from build123d import *

# Parameters (mm, degrees)
F1_DEPTH = 65
F2_DEPTH = 14
F3_DEPTH = 14
F4_R     = 1
F5_DEPTH = 14


# Not quite as in the source:
# - a feature names something its author has since deleted; it is built from what else it names


with BuildPart() as f1:
    # F0 (on Top) → F1 (new body)
    with BuildSketch(Plane.XY):
        with BuildLine():
            ThreePointArc((0, -3), (2.1213203436, -2.1213203436), (3, 0))
            Line((3, 0), (0, 0))
            Line((0, 0), (0, -3))
        make_face()
        with BuildLine():
            Line((0, 0), (3, 0))
            ThreePointArc((3, 0), (2.1213203436, 2.1213203436), (0, 3))
            Line((0, 3), (0, 0))
        make_face()
        with BuildLine():
            Line((0, 0), (0, 3))
            ThreePointArc((0, 3), (-2.1213203436, 2.1213203436), (-3, 0))
            Line((-3, 0), (0, 0))
        make_face()
        with BuildLine():
            ThreePointArc((-3, 0), (-2.1213203436, -2.1213203436), (0, -3))
            Line((0, -3), (0, 0))
            Line((0, 0), (-3, 0))
        make_face()
    extrude(amount=F1_DEPTH)



with BuildPart() as f2:
    # F0 (on Top) → F2 (new body)
    with BuildSketch(Plane.XY):
        with BuildLine():
            ThreePointArc((-4.8989794856, 3), (-3.8729833462, 7.1622776602), (0, 9))
            Line((0, 9), (0, 12.5))
            ThreePointArc((0, 12.5), (-0.545120999, 12.4881080671), (-1.0892047912, 12.4524548954))
            ThreePointArc((-1.0892047912, 12.4524548954), (-8.8388347648, 8.8388347648), (-12.4524548954, 1.0892047912))
            ThreePointArc((-12.4524548954, 1.0892047912), (-12.4881080671, 0.545120999), (-12.5, 0))
            Line((-12.5, 0), (-4.8989794856, 0))
            Line((-4.8989794856, 0), (-4.8989794856, 3))
        make_face()
        with BuildLine():
            Line((0, -12.5), (0, -9))
            ThreePointArc((0, -9), (-3.8729833462, -7.1622776602), (-4.8989794856, -3))
            Line((-4.8989794856, -3), (-4.8989794856, 0))
            Line((-4.8989794856, 0), (-12.5, 0))
            ThreePointArc((-12.5, 0), (-8.8388347648, -8.8388347648), (0, -12.5))
        make_face()
        with BuildLine():
            Line((12.5, 0), (4.8989794856, 0))
            Line((4.8989794856, 0), (4.8989794856, -3))
            ThreePointArc((4.8989794856, -3), (3.8729833462, -7.1622776602), (0, -9))
            Line((0, -9), (0, -12.5))
            ThreePointArc((0, -12.5), (0.545120999, -12.4881080671), (1.0892047912, -12.4524548954))
            ThreePointArc((1.0892047912, -12.4524548954), (8.8388347648, -8.8388347648), (12.4524548954, -1.0892047912))
            ThreePointArc((12.4524548954, -1.0892047912), (12.4881080671, -0.545120999), (12.5, 0))
        make_face()
        with BuildLine():
            Line((4.8989794856, 3), (4.8989794856, 0))
            Line((4.8989794856, 0), (12.5, 0))
            ThreePointArc((12.5, 0), (8.8388347648, 8.8388347648), (0, 12.5))
            Line((0, 12.5), (0, 9))
            ThreePointArc((0, 9), (3.8729833462, 7.1622776602), (4.8989794856, 3))
        make_face()
    extrude(amount=F2_DEPTH)


with BuildPart() as f1_1:
    add(f1.part)

    add(f2.part)  # F2#2 merges F2
    # F0 (on Top) → F2, piece 2 (join)
    with BuildSketch(Plane.XY):
        with BuildLine():
            ThreePointArc((-3, 0), (-2.1213203436, 2.1213203436), (0, 3))
            Line((0, 3), (-4.8989794856, 3))
            ThreePointArc((-4.8989794856, 3), (-4.2247448714, 1.3257653858), (-3, 0))
        make_face()
        with BuildLine():
            ThreePointArc((0, 3), (2.1213203436, 2.1213203436), (3, 0))
            ThreePointArc((3, 0), (4.2247448714, 1.3257653858), (4.8989794856, 3))
            Line((4.8989794856, 3), (0, 3))
        make_face()
        with BuildLine():
            ThreePointArc((4.8989794856, -3), (4.2247448714, -1.3257653858), (3, 0))
            ThreePointArc((3, 0), (2.1213203436, -2.1213203436), (0, -3))
            Line((0, -3), (4.8989794856, -3))
        make_face()
        with BuildLine():
            Line((-4.8989794856, -3), (0, -3))
            ThreePointArc((0, -3), (-2.1213203436, -2.1213203436), (-3, 0))
            ThreePointArc((-3, 0), (-4.2247448714, -1.3257653858), (-4.8989794856, -3))
        make_face()
    extrude(amount=F2_DEPTH)

    # F0 (on Top) → F3 (join)
    with BuildSketch(Plane.XY):
        with BuildLine():
            Line((20, 0), (12.5, 0))
            ThreePointArc((12.5, 0), (14.2975101103, -0.811390688), (16.25, -1.0892047912))
            ThreePointArc((16.25, -1.0892047912), (18.2024898897, -0.811390688), (20, 0))
        make_face()
        with BuildLine():
            ThreePointArc((-1.0892047912, 16.25), (-0.811390688, 14.2975101103), (0, 12.5))
            Line((0, 12.5), (0, 20))
            ThreePointArc((0, 20), (-0.811390688, 18.2024898897), (-1.0892047912, 16.25))
        make_face()
        with BuildLine():
            Line((-20, 0), (-12.5, 0))
            ThreePointArc((-12.5, 0), (-14.2975101103, 0.811390688), (-16.25, 1.0892047912))
            ThreePointArc((-16.25, 1.0892047912), (-18.2024898897, 0.811390688), (-20, 0))
        make_face()
        with BuildLine():
            ThreePointArc((1.0892047912, -16.25), (0.811390688, -14.2975101103), (0, -12.5))
            Line((0, -12.5), (0, -20))
            ThreePointArc((0, -20), (0.811390688, -18.2024898897), (1.0892047912, -16.25))
        make_face()
        with BuildLine():
            ThreePointArc((16.25, -1.0892047912), (14.2975101103, -0.811390688), (12.5, 0))
            ThreePointArc((12.5, 0), (12.4881080671, -0.545120999), (12.4524548954, -1.0892047912))
            Line((12.4524548954, -1.0892047912), (16.25, -1.0892047912))
        make_face()
        with BuildLine():
            ThreePointArc((-1.0892047912, 12.4524548954), (-0.545120999, 12.4881080671), (0, 12.5))
            ThreePointArc((0, 12.5), (-0.811390688, 14.2975101103), (-1.0892047912, 16.25))
            Line((-1.0892047912, 16.25), (-1.0892047912, 12.4524548954))
        make_face()
        with BuildLine():
            ThreePointArc((-16.25, 1.0892047912), (-14.2975101103, 0.811390688), (-12.5, 0))
            ThreePointArc((-12.5, 0), (-12.4881080671, 0.545120999), (-12.4524548954, 1.0892047912))
            Line((-12.4524548954, 1.0892047912), (-16.25, 1.0892047912))
        make_face()
        with BuildLine():
            ThreePointArc((1.0892047912, -12.4524548954), (0.545120999, -12.4881080671), (0, -12.5))
            ThreePointArc((0, -12.5), (0.811390688, -14.2975101103), (1.0892047912, -16.25))
            Line((1.0892047912, -16.25), (1.0892047912, -12.4524548954))
        make_face()
    extrude(amount=F3_DEPTH)

    # F4
    f4_edges = [f1_1.edges().sort_by_distance(p)[0] for p in [
        (3, 0, 65),
    ]]
    fillet(f4_edges, radius=F4_R)

    # F0 (on Top) → F5 (join)
    with BuildSketch(Plane.XY):
        with BuildLine():
            ThreePointArc((-4.8989794856, -3), (-4.2247448714, -1.3257653858), (-3, 0))
            Line((-3, 0), (-4.8989794856, 0))
            Line((-4.8989794856, 0), (-4.8989794856, -3))
        make_face()
        with BuildLine():
            Line((-4.8989794856, 0), (-3, 0))
            ThreePointArc((-3, 0), (-4.2247448714, 1.3257653858), (-4.8989794856, 3))
            Line((-4.8989794856, 3), (-4.8989794856, 0))
        make_face()
        with BuildLine():
            ThreePointArc((4.8989794856, 3), (4.2247448714, 1.3257653858), (3, 0))
            Line((3, 0), (4.8989794856, 0))
            Line((4.8989794856, 0), (4.8989794856, 3))
        make_face()
        with BuildLine():
            Line((4.8989794856, 0), (3, 0))
            ThreePointArc((3, 0), (4.2247448714, -1.3257653858), (4.8989794856, -3))
            Line((4.8989794856, -3), (4.8989794856, 0))
        make_face()
    extrude(amount=F5_DEPTH)


solid = f1_1.part
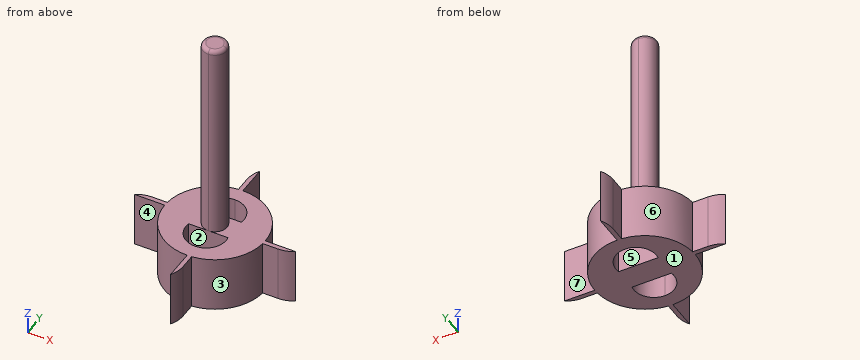
Work out the finished part from the listing and answer in its coordinate system (mm). Face numbers are marked on the shaded views. A direction names the side the tool comes from. Round coordinates to 2 decimals unless told otherwise and drop trailing zeros. Loops run counter-clockwise (first coordinate to the right, second up) from the corner with the lowest first, then second, coordinate; pieces in that order, holes last. Notation, with made-up numbers: (3, 12) -> (44, 12) arc R14 cw to (44, 18) -> close; hole circle Ø11 at (70.5, 77). An arc over 180 degrees is marked (long way). Use one line per item in the form item = value.
(1) Find section C-C on x = -14. Give the vertices of the cut face in (y, z).
Answer list:
outline = (0, 0) -> (1.09, 0) -> (1.09, 14) -> (0, 14) -> close
(2) For a pull along Y with two mould halves and no side action, classify the marked faces 1, 2 and 3 as released by +Y, released by -Y, zero draft, split by the parting line, or undercut.
Answer list:
face_1 = zero draft
face_2 = undercut
face_3 = released by -Y
(3) A tool of negligible diameter and unlimited length cuts with its end or side. For the marked faces 4, 5, 6 and 7, from which of +Z, -Z, +X, -X, +Y, -Y can it reach the whole face along a straight path? Write none if from no direction.
Answer list:
face_4 = +Z, -Z, -X, -Y
face_5 = +Z, -Z
face_6 = +Z, -Z, -X, +Y
face_7 = +Z, -Z, +X, +Y
(4) Find section D-D on z = 33.5. Give the vertices of the cut face in (x, y), then the cut area to 3 significant figures.
Answer list:
outline = circle Ø6 at (0, 0)
area = 28.3 mm2
(5) Find section A-A on z = 5.5. Give the vertices of the cut face in (x, y), then the cut area to 3 significant figures.
Answer list:
outline = (-20, 0) -> (-12.5, 0) arc R12.5 ccw to (0, -12.5) -> (0, -20) arc R7 ccw to (1.09, -16.25) -> (1.09, -12.45) arc R12.5 ccw to (12.45, -1.09) -> (16.25, -1.09) arc R7 ccw to (20, 0) -> (12.5, 0) arc R12.5 ccw to (0, 12.5) -> (0, 20) arc R7 ccw to (-1.09, 16.25) -> (-1.09, 12.45) arc R12.5 ccw to (-12.45, 1.09) -> (-16.25, 1.09) arc R7 ccw to start; hole (-4.9, -3) arc R5 ccw (long way) to (4.9, -3) -> close; hole (-4.9, 3) -> (4.9, 3) arc R5 ccw (long way) to start
area = 420 mm2
(6) Flat-ended cylindrical pins translate along their axes: P1, Ø8, axis at y = 17, z = 6.5, coming from the +X side; P2, Ø1.9, axis at x = 15, z = 3.5, coming from the -Y side; P3, Ø2, axis at x = 17.5, z = 10, coming from the +Y side. Find the tip coordinate at first contact, or state that the pin passes through.
Answer list:
P1 = 0
P2 = -1.09
P3 = 0
(7) Find section B-B on y = -5. Give the vertices of the cut face in (x, z), then the cut area to 3 significant figures.
Answer list:
outline = (-11.46, 0) -> (-4.9, 0) -> (-4.9, 14) -> (-11.46, 14) -> close; (4.9, 0) -> (11.46, 0) -> (11.46, 14) -> (4.9, 14) -> close
area = 184 mm2
(8) Straight lines are drawn through the part: line 1 (Z direction, x = 7, y = 4.5); line 2 (Y direction, x = 13, z = 13.5); line 3 (X direction, y = -2, z = 17). For each, find the intervals that lie inside material, in ascending order.
Answer list:
line_1 = 0 to 14
line_2 = -1.09 to 0
line_3 = -2.24 to 2.24
